Could you check a few things on this model? Use its own coordinates, in mm. Face numbers are marked on the shaded views. Round coordinates to 2 decimals unless told otherwise and drop trailing zeros. Write each loop counter-clockwise with the first axis right and the second up, starting at its lowest first coordinate (ties: lowest second). Pieces come first, ordered by that corner, then holes. Notation, with made-up numbers: (-31.75, 74) - (-22.75, 74) arc R22 cw to (-22.75, 112) - close; hole circle Ø6 at (-2, -7.5). An arc over 180 degrees is marked (long way). Write each question's results on one line, items separated by ' | '. Start each with the question number.
(1) For P1, Ø6, axis at x = -19.5, z = 3.5, coming from the -Y side; P2, Ø7.5, axis at x = -19.05, z = 0, coming from the +Y side (3 decimals); P3, Ø4, axis at x = 17.5, z = 5, coming from the -Y side, each with a flat end and sliding along its axis, tell me the tip position at first contact or that it passes through.
(2) Imagine slicing it at C-C on x = -19.05. State how many separate pieces and enclosed holes the cut face has, then the cut area to 3 significant figures.
(3) Please list where these lines run through material, in increasing order: line 1 (Y direction, x = -3, z = 0) (3 decimals); line 2 (Z direction, x = -19, y = 6.75); line 3 (X direction, y = -9.1, z = 0). Write a range as [from, to].
(4) Thinking about a two-plate mould opening in Y: for the marked faces 1 and 2, which applies, +Y half, -Y half, draft (parallel to the pull), parting line (faces both ways), or undercut?
(5) Imagine slicing it at A-A on y = 0. Write out the boundary of the cut face in (x, z) (3 decimals).
(6) Imagine slicing it at B-B on z = 0. Write out the boundary of the cut face in (x, y) (3 decimals), then the cut area to 3 significant figures.
(7) Imagine slicing it at D-D on z = -4. Write out the boundary of the cut face in (x, y), then the cut area to 3 significant figures.
```python
from build123d import *

# Parameters (mm, degrees)
SKETCH1_R          = 9.525
SKETCH1_R_2        = 8.2804
EXTRUDE1_DEPTH     = 25.4
SKETCH2_R          = 2.38125
CUT_EXTRUDE1_DEPTH = 29.750847814
CIRPATTERN1_COUNT  = 3
CIRPATTERN1_ANGLE  = 120


with BuildPart() as part:
    # Sketch1 → Extrude1 (new, symmetric)
    with BuildSketch(Plane(origin=(0, 0, 0), x_dir=(0, 0, -1), z_dir=(1, 0, 0))):
        Circle(SKETCH1_R)
        Circle(SKETCH1_R_2, mode=Mode.SUBTRACT)
    extrude(amount=EXTRUDE1_DEPTH, both=True)

    # Sketch2 → Cut-Extrude1 (cut, symmetric)
    with BuildSketch(Plane(origin=(0, 0, 0), x_dir=(1, 0, 0), z_dir=(0, 1, 0))):
        with Locations(Location((-19.05, 0, 0), (0, 0, 270))):
            Circle(SKETCH2_R)
    cut_extrude1 = extrude(amount=CUT_EXTRUDE1_DEPTH, both=True, mode=Mode.SUBTRACT)

    # CirPattern1: Cut-Extrude1 ×3 about axis
    cirpattern1_axis = Axis((25.4, 0, 0), (-1, 0, 0))
    for i in range(1, CIRPATTERN1_COUNT):
        add(cut_extrude1.rotate(cirpattern1_axis, i * CIRPATTERN1_ANGLE / (CIRPATTERN1_COUNT - 1)), mode=Mode.SUBTRACT)


solid = part.part
```
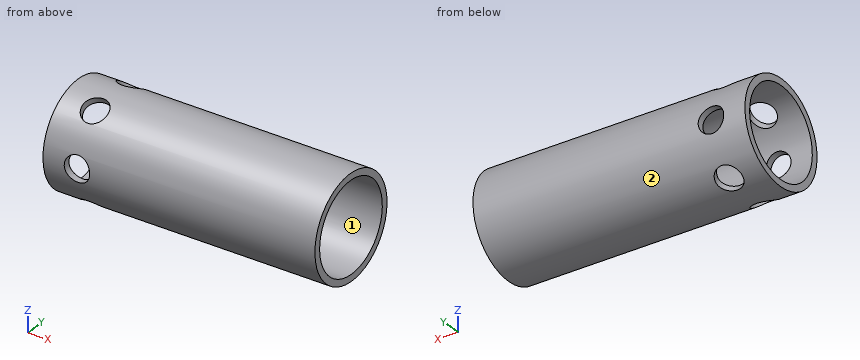
Response:
1) P1: y = -9.47 | P2: y = 9.525 | P3: y = -9.04
2) separate pieces: 6 | enclosed holes: 0 | area: 33.6 mm²
3) line 1: [-9.525, -8.28], [8.28, 9.525] | line 2: [-6.72, -4.8], [4.8, 6.72] | line 3: [-25.4, -21.43], [-16.67, 25.4]
4) face 1: undercut | face 2: parting line
5) outline: (-25.4, -9.525) - (25.4, -9.525) - (25.4, -8.28) - (-25.4, -8.28) - close; (-25.4, 8.28) - (25.4, 8.28) - (25.4, 9.525) - (-25.4, 9.525) - close
6) outline: (-25.4, -9.525) - (-21.431, -9.525) - (-21.431, -8.28) - (-25.4, -8.28) - close; (-25.4, 8.28) - (-21.431, 8.28) - (-21.431, 9.525) - (-25.4, 9.525) - close; (-16.669, -9.525) - (25.4, -9.525) - (25.4, -8.28) - (-16.669, -8.28) - close; (-16.669, 8.28) - (25.4, 8.28) - (25.4, 9.525) - (-16.669, 9.525) - close | area: 115 mm²
7) outline: (-25.4, -8.64) - (25.4, -8.64) - (25.4, -7.25) - (-25.4, -7.25) - close; (-25.4, 7.25) - (25.4, 7.25) - (25.4, 8.64) - (-25.4, 8.64) - close | area: 142 mm²
